For this review, take the finished solid that the model builds, in its own axes (mm). Face numbers are marked on the shaded views. A direction names the side the tool comes from. Round coordinates to 2 decimals unless told otherwise and drop trailing zeros. Order: outer loops, then holes, each group sorted by start corner. A loop starts at its lowest first (then second) coordinate and runs counter-clockwise, first axis right, second up. Notation, with made-up numbers: (29.5, 51.5) -> (47.5, 51.5) arc R29 cw to (47.5, 73.5) -> close; hole circle Ø7 at (84.5, 25.25). An arc over 180 degrees is marked (long way). Answer in a Markdown table with one row per item.
Autodesk Inventor part; units mm, degrees
ref_plane "YZ Plane" through (0, 0, 0) normal (1, 0, 0) x (0, 1, 0)
ref_plane "XZ Plane" through (0, 0, 0) normal (0, 1, 0) x (-1, 0, 0)
ref_plane "XY Plane" through (0, 0, 0) normal (0, 0, 1) x (1, 0, 0)
sketch "Boceto1" plane through (0, 0, 0) normal (0, 0, 1) x (1, 0, 0)
  circle A0 centre (0, 0) radius 20
  circle A1 centre (0, 0) radius 18
  dimension "d0" = 40
  dimension "d1" = 36
extrude "Extrusión1" add sketch "Boceto1" along normal blind 4
sketch "Boceto2" plane through (0, 0, 0) normal (0, 0, -1) x (-1, 0, 0)
  circle A0 centre (0, 0) radius 16
  circle A1 centre (0, 0) radius 14
  circle A2 centre (0, 0) radius 12
  circle A3 centre (0, 0) radius 10
  circle A4 centre (0, 0) radius 8
  circle A5 centre (0, 0) radius 6
  circle A6 centre (0, 0) radius 4
  dimension "d4" = 32
  dimension "d5" = 28
  dimension "d6" = 24
  dimension "d7" = 20
  dimension "d8" = 16
  dimension "d9" = 12
  dimension "d10" = 8
extrude "Extrusión2" add sketch "Boceto2" against normal blind 2
sketch "Boceto3" plane through (0, 0, 0) normal (0, 0, -1) x (-1, 0, 0)
  line L0 (-19.4045, 1) -> (19.4045, 1)
  line L1 (19.4045, 1) -> (19.4045, -1)
  line L2 (19.4045, -1) -> (-19.4045, -1)
  line L3 (-19.4045, -1) -> (-19.4045, 1)
  line L4 (-19.4045, 1) -> (19.4045, -1) construction
  line L5 (19.4045, 1) -> (-19.4045, -1) construction
  line L6 (-1, 19.4045) -> (1, 19.4045)
  line L7 (1, 19.4045) -> (1, -19.4045)
  line L8 (1, -19.4045) -> (-1, -19.4045)
  line L9 (-1, -19.4045) -> (-1, 19.4045)
  line L10 (-1, 19.4045) -> (1, -19.4045) construction
  line L11 (1, 19.4045) -> (-1, -19.4045) construction
  point P0 (0, 0)
  point P1 (0, 0)
  dimension "d13" = 2
  dimension "d14" = 2
extrude "Extrusión3" add sketch "Boceto3" against normal blind 2
equation "\"Radio_pliegue\" = Grosor"
equation "\"Anchura_desahogo_plegado\" = Grosor"
equation "\"Profundidad_desahogo_plegado\" = 0.5 * Grosor"
equation "\"Tamaño_destalonado\" = 4 * Grosor"
equation "\"Remanente_mínimo\" = 2 * Grosor"
equation "\"Radiodetransición\" = Radio_pliegue"
equation "\"Tamaño_de_radio_de_Jacobi\" = Radio_pliegue"
equation "\"TamañoSeparación\" = Grosor"
properties part number "Lattice bottom"
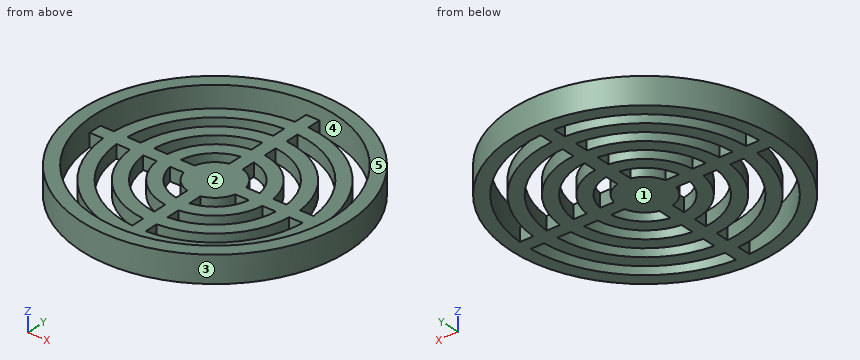
Q1. Clearance check with flat-ended pins moving along their axes: pin 1 Ø0.6 at (y, z) = (-12.5, 1) entering from +X; pin 2 Ø2 at (y, z) = (-16.5, 0.5) entering from -X; pin 3 Ø0.6 at (x, z) = (4.5, 1) entering from -Y. State where each tip first meets the part, or that it passes through.
Answer key:
| item | result |
|---|---|
| pin 1 | stops at x = 15.85 |
| pin 2 | stops at x = -12.64 |
| pin 3 | stops at y = -19.55 |
Q2. Take a section at B-B, the plane y = 13. Write out the cut boundary in (x, z).
Answer key:
| item | result |
|---|---|
| outline | (-15.2, 0) -> (-12.45, 0) -> (-12.45, 4) -> (-15.2, 4) -> close; (-9.33, 0) -> (-5.2, 0) -> (-5.2, 2) -> (-9.33, 2) -> close; (-1, 0) -> (1, 0) -> (1, 2) -> (-1, 2) -> close; (5.2, 0) -> (9.33, 0) -> (9.33, 2) -> (5.2, 2) -> close; (12.45, 0) -> (15.2, 0) -> (15.2, 4) -> (12.45, 4) -> close |
Q3. Take a section at A-A, the plane x = 0. Write out the cut boundary in (y, z).
Answer key:
| item | result |
|---|---|
| outline | (-20, 0) -> (20, 0) -> (20, 4) -> (18, 4) -> (18, 2) -> (-18, 2) -> (-18, 4) -> (-20, 4) -> close |
Q4. The part is to be moulded in two halves that separate along X. For the marked faces 3, 4 and 5, say which applies: +X half, -X half, draft (parallel to the pull), parting line (faces both ways), or undercut.
Answer key:
| item | result |
|---|---|
| face 3 | parting line |
| face 4 | undercut |
| face 5 | draft |
Q5. Take a section at C-C, the plane y = -9. Write out the cut boundary in (x, z).
Answer key:
| item | result |
|---|---|
| outline | (-17.86, 0) -> (-15.59, 0) -> (-15.59, 4) -> (-17.86, 4) -> close; (-13.23, 0) -> (-10.72, 0) -> (-10.72, 2) -> (-13.23, 2) -> close; (-7.94, 0) -> (-4.36, 0) -> (-4.36, 2) -> (-7.94, 2) -> close; (-1, 0) -> (1, 0) -> (1, 2) -> (-1, 2) -> close; (4.36, 0) -> (7.94, 0) -> (7.94, 2) -> (4.36, 2) -> close; (10.72, 0) -> (13.23, 0) -> (13.23, 2) -> (10.72, 2) -> close; (15.59, 0) -> (17.86, 0) -> (17.86, 4) -> (15.59, 4) -> close |
Q6. Tool access review of the marked faces 1 and 2: name each direction out of +Z, -Z, +X, -X, +Y, -Y from which nothing blocks a thin tool from reaching the whole face with its end or side.
Answer key:
| item | result |
|---|---|
| face 1 | -Z, +X, -X, +Y, -Y |
| face 2 | +Z |
Q7. Take a section at D-D, the plane z = 2.5. Write out the cut boundary in (x, y).
Answer key:
| item | result |
|---|---|
| outline | circle Ø40 at (0, 0); hole circle Ø36 at (0, 0) |
Q8. To check wall thickness, follow probe 1 along Y at (x, z) = (0, 2.3); probe 2 along Z at (x, y) = (14.5, 4); probe 3 along Y at (x, z) = (9, 3.55). State the ranges of each line that lie inside material, in increasing order.
Answer key:
| item | result |
|---|---|
| probe 1 | y = -20 to -18, 18 to 20 |
| probe 2 | z = 0 to 2 |
| probe 3 | y = -17.86 to -15.59, 15.59 to 17.86 |
